from build123d import *

# Parameters (mm, degrees)
SKETCH1_W           = 25.4
SKETCH1_H           = 50.8
SKETCH1_W_2         = 20.32
SKETCH1_H_2         = 45.72
BOSS_EXTRUDE1_DEPTH = 304.8
SKETCH2_R           = 3.175
CUT_EXTRUDE1_DEPTH  = 304.8


with BuildPart() as part:
    # Sketch1 → Boss-Extrude1 (new body)
    with BuildSketch(Plane(origin=(0, 0, 0), x_dir=(0, 0, -1), z_dir=(1, 0, 0))):
        Rectangle(SKETCH1_W, SKETCH1_H)
        Rectangle(SKETCH1_W_2, SKETCH1_H_2, mode=Mode.SUBTRACT)
    extrude(amount=BOSS_EXTRUDE1_DEPTH)

    # Sketch2 → Cut-Extrude1 (cut)
    with BuildSketch(Plane(origin=(0, 25.4, 0), x_dir=(1, 0, 0), z_dir=(0, 1, 0))):
        with Locations(Location((12.7, 0, 0), (0, 0, 270))):
            Circle(SKETCH2_R)
        with Locations(Location((38.1, 0, 0), (0, 0, 270))):
            Circle(SKETCH2_R)
        with Locations(Location((63.5, 0, 0), (0, 0, 270))):
            Circle(SKETCH2_R)
        with Locations(Location((88.9, 0, 0), (0, 0, 270))):
            Circle(SKETCH2_R)
        with Locations(Location((114.3, 0, 0), (0, 0, 270))):
            Circle(SKETCH2_R)
        with Locations(Location((139.7, 0, 0), (0, 0, 270))):
            Circle(SKETCH2_R)
        with Locations(Location((165.1, 0, 0), (0, 0, 270))):
            Circle(SKETCH2_R)
        with Locations(Location((190.5, 0, 0), (0, 0, 270))):
            Circle(SKETCH2_R)
        with Locations(Location((215.9, 0, 0), (0, 0, 270))):
            Circle(SKETCH2_R)
        with Locations(Location((241.3, 0, 0), (0, 0, 270))):
            Circle(SKETCH2_R)
        with Locations(Location((266.7, 0, 0), (0, 0, 270))):
            Circle(SKETCH2_R)
        with Locations(Location((292.1, 0, 0), (0, 0, 270))):
            Circle(SKETCH2_R)
    extrude(amount=-CUT_EXTRUDE1_DEPTH, mode=Mode.SUBTRACT)


solid = part.part
Work out the finished part from the listing and answer in its coordinate system (mm). A direction names the side the tool comes from. Coordinates: 2 decimals unless noted, no trailing zeros. Write each loop counter-clockwise with the first axis right and the second up, starting at its lowest first coordinate (ties: lowest second). Pieces come first, ordered by that corner, then holes. Notation, with made-up numbers: M 77.25,37 L 131.25,37 A14 ccw 131.25,41 Z; hole C -39.5,-2 d2. An arc over 180 degrees is marked long. Write item = value, one per line.
1. For faces 4 (the face through (85.8, 24.15, -0.69)), 5 (the face through (150, -22.86, 0)), determine the directions among +Z, -Z, +X, -X, +Y, -Y from which every point of the face is accessible in a straight line to the end or side of a thin tool.
Solution:
face_4 = +Y, -Y
face_5 = +X, -X
2. Determine the mould class of faces 1 (the face through (150, 0, -12.7)), 2 (the face through (150, 0, -10.16)), 3 (the face through (0, 2, 10.4)) for opening direction Z: released by +Z, released by -Z, zero draft, split by the parting line, or undercut.
Solution:
face_1 = released by -Z
face_2 = undercut
face_3 = zero draft
3. The part is cut by section B-B (y = 5). Determine the outline of the cut face in (x, z), then the cut area to 3 significant figures.
Solution:
outline = M 0,-12.7 L 304.8,-12.7 L 304.8,-10.16 L 0,-10.16 Z; M 0,10.16 L 304.8,10.16 L 304.8,12.7 L 0,12.7 Z
area = 1,550 mm2
4. The part is cut by section C-C (x = 88.9). Determine the outline of the cut face in (y, z) (3 decimals).
Solution:
outline = M -25.4,-12.7 L 25.4,-12.7 L 25.4,-3.175 L 22.86,-3.175 L 22.86,-10.16 L -22.86,-10.16 L -22.86,-3.175 L -25.4,-3.175 Z; M -25.4,3.175 L -22.86,3.175 L -22.86,10.16 L 22.86,10.16 L 22.86,3.175 L 25.4,3.175 L 25.4,12.7 L -25.4,12.7 Z
5. Straight lines are drawn through the part: line 1 (Z direction, x = 221.5, y = -16); line 2 (Y direction, x = 147, z = 7.25); line 3 (Z direction, x = 215.9, y = 23.7) (3 decimals). For each, find the intervals that lie inside material, in ascending order. Write a range as from..to.
Solution:
line_1 = -12.7..-10.16, 10.16..12.7
line_2 = -25.4..-22.86, 22.86..25.4
line_3 = -12.7..-3.175, 3.175..12.7
6. The part is cut by section A-A (z = -6.5). Determine the outline of the cut face in (x, y).
Solution:
outline = M 0,-25.4 L 304.8,-25.4 L 304.8,-22.86 L 0,-22.86 Z; M 0,22.86 L 304.8,22.86 L 304.8,25.4 L 0,25.4 Z
